from build123d import *

# Parameters (mm, degrees)
SKETCH1_R           = 37.5
BOSS_EXTRUDE1_DEPTH = 4
SKETCH4_R           = 1.5
BOSS_EXTRUDE2_DEPTH = 2
SKETCH5_R           = 2
CUT_EXTRUDE2_DEPTH  = 10
SKETCH6_R           = 4.75
CUT_EXTRUDE3_DEPTH  = 42


with BuildPart() as part:
    # Sketch1 → Boss-Extrude1 (new body)
    with BuildSketch(Plane(origin=(0, 0, 0), x_dir=(1, 0, 0), z_dir=(0, 1, 0))):
        Circle(SKETCH1_R)
    extrude(amount=BOSS_EXTRUDE1_DEPTH)

    # Sketch4 → Boss-Extrude2 (add)
    with BuildSketch(Plane(origin=(0, 4, 0), x_dir=(1, 0, 0), z_dir=(0, 1, 0))):
        with Locations((0, 32)):
            Circle(SKETCH4_R)
        with Locations((16, 27.712812921)):
            Circle(SKETCH4_R)
        with Locations((27.712812921, 16)):
            Circle(SKETCH4_R)
        with Locations((32, 0)):
            Circle(SKETCH4_R)
        with Locations((27.712812921, -16)):
            Circle(SKETCH4_R)
        with Locations((16, -27.712812921)):
            Circle(SKETCH4_R)
        with Locations((0, -32)):
            Circle(SKETCH4_R)
        with Locations((-16, -27.712812921)):
            Circle(SKETCH4_R)
        with Locations((-27.712812921, -16)):
            Circle(SKETCH4_R)
        with Locations((-32, 0)):
            Circle(SKETCH4_R)
        with Locations((-27.712812921, 16)):
            Circle(SKETCH4_R)
        with Locations((-16, 27.712812921)):
            Circle(SKETCH4_R)
    extrude(amount=BOSS_EXTRUDE2_DEPTH)

    # Sketch5 → Cut-Extrude2 (cut)
    with BuildSketch(Plane(origin=(0, 4, 0), x_dir=(1, 0, 0), z_dir=(0, 1, 0))):
        with Locations((-17.5, -8)):
            Circle(SKETCH5_R)
        with Locations((17.5, -8)):
            Circle(SKETCH5_R)
    extrude(amount=-CUT_EXTRUDE2_DEPTH, mode=Mode.SUBTRACT)

    # Sketch6 → Cut-Extrude3 (cut)
    with BuildSketch(Plane(origin=(0, 4, 0), x_dir=(1, 0, 0), z_dir=(0, 1, 0))):
        Circle(SKETCH6_R)
    extrude(amount=-CUT_EXTRUDE3_DEPTH, mode=Mode.SUBTRACT)


solid = part.part
Could you check a few things on this model? Use its own coordinates, in mm. A direction names the side the tool comes from. Give positions to 0.01 mm unless a question says otherwise; leave off trailing zeros. Order: outer loops, then holes, each group sorted by start corner. A loop starts at its lowest first (then second) coordinate and runs counter-clockwise, first axis right, second up. Notation, with made-up numbers: (26.5, -23.5) -> (59.5, -23.5) arc R14 cw to (59.5, 2.5) -> close; hole circle Ø9 at (14.25, -12.5). An arc over 180 degrees is marked (long way). Return JSON: item names as keys, results as strings.
1. Imagine slicing it at C-C on z = 8. List the corners of the cut face in (x, y) for me, then the cut area to 3 significant figures.
Answer list:
{"outline": "(-36.64, 0) -> (-19.5, 0) -> (-19.5, 4) -> (-36.64, 4) -> close; (-15.5, 0) -> (15.5, 0) -> (15.5, 4) -> (-15.5, 4) -> close; (19.5, 0) -> (36.64, 0) -> (36.64, 4) -> (19.5, 4) -> close", "area": "261 mm2"}
2. For pin 1 Ø5 at (x, z) = (-17.5, 8) entering from +Y; pin 2 Ø5 at (x, z) = (17.5, 8) entering from -Y; pin 3 Ø2 at (x, y) = (-22, 1) entering from -Z; pin 4 Ø1.5 at (x, y) = (-2.5, 5.5) entering from +Z, each with a flat end and sliding along its axis, tell me the tip position at first contact or that it passes through.
Answer list:
{"pin 1": "stops at y = 4", "pin 2": "stops at y = 0", "pin 3": "stops at z = -31.07", "pin 4": "passes through"}
3. Imagine slicing it at A-A on z = 0. List the corners of the cut face in (x, y) for me, then the cut area to 3 significant figures.
Answer list:
{"outline": "(-37.5, 0) -> (-4.75, 0) -> (-4.75, 4) -> (-30.5, 4) -> (-30.5, 6) -> (-33.5, 6) -> (-33.5, 4) -> (-37.5, 4) -> close; (4.75, 0) -> (37.5, 0) -> (37.5, 4) -> (33.5, 4) -> (33.5, 6) -> (30.5, 6) -> (30.5, 4) -> (4.75, 4) -> close", "area": "274 mm2"}
4. Thinking about a two-plate mould opening in X: for faces 3 (the cylindrical face through (-1.2, 5, 32.9)), 4 (the flat face through (-16, 6, -28)), 5 (the cylindrical face through (16.026, 2.028, 6.648)), 6 (the cylindrical face through (-17.5, 4.99, -27.78)), which applies, pulls with the +X half, pulls with the -X half, needs draft (parallel to the pull), parting line crosses it, or undercut?
Answer list:
{"face 3": "parting line crosses it", "face 4": "needs draft", "face 5": "undercut", "face 6": "undercut"}
5. Imagine slicing it at D-D on x = 32. List the corners of the cut face in (y, z) for me, then the cut area to 3 significant figures.
Answer list:
{"outline": "(0, -19.55) -> (4, -19.55) -> (4, -1.5) -> (6, -1.5) -> (6, 1.5) -> (4, 1.5) -> (4, 19.55) -> (0, 19.55) -> close", "area": "162 mm2"}
6. On a 3-axis mill with a long thin cutter (end or side, diameter ignored), from which of +Z, -Z, +X, -X, +Y, -Y can I reach the whole of each face in a straight line? I mean faces 1 (the cylindrical face through (14.81, 4.99, -26.8)), 2 (the flat face through (-32, 6, 0)). Say none if no direction works.
Answer list:
{"face 1": "+Y", "face 2": "+Z, -Z, +X, -X, +Y"}
7. I need wall thicknesses on line 1 (X direction, y = 2.35, z = 8); line 2 (Y direction, x = 14.5, z = 9); line 3 (Z direction, x = 0, y = 2.55). Which ranges of each line are inside material? Lowest first, please. Write a range as from..to.
Answer list:
{"line 1": "x = -36.64..-19.5, -15.5..15.5, 19.5..36.64", "line 2": "y = 0..4", "line 3": "z = -37.5..-4.75, 4.75..37.5"}
8. Imagine slicing it at B-B on y = 1.9. List the corners of the cut face in (x, z) for me, then the cut area to 3 significant figures.
Answer list:
{"outline": "circle Ø75 at (0, 0); hole circle Ø4 at (-17.5, 8); hole circle Ø9.5 at (0, 0); hole circle Ø4 at (17.5, 8)", "area": "4,320 mm2"}
